from build123d import *

# Parameters (mm, degrees)
SKETCH_R        = 11.3
SKETCH_R_2      = 1.6
SKETCH_R_3      = 3.2
PAD_DEPTH       = 15
SKETCH001_R     = 3.2
POCKET_DEPTH    = 3.4
SKETCH002_R     = 6.1
POCKET001_DEPTH = 4
FILLET_R        = 4
FILLET001_R     = 4
CHAMFER_SIZE    = 0.6
CHAMFER001_SIZE = 0.6
CHAMFER002_SIZE = 0.6


with BuildPart() as part:
    # Sketch → Pad (new body)
    with BuildSketch(Plane.XY):
        Polygon((20, 30), (20, 58), (62.3, 58), (62.3, 30), (82.3, 30), (82.3, 0), (0, 0), (0, 30), align=None)
        with Locations((41.15, 36.85)):
            Circle(SKETCH_R, mode=Mode.SUBTRACT)
        with Locations((25.65, 52.35)):
            Circle(SKETCH_R_2, mode=Mode.SUBTRACT)
        with Locations((25.65, 21.35)):
            Circle(SKETCH_R_2, mode=Mode.SUBTRACT)
        with Locations((56.65, 52.35)):
            Circle(SKETCH_R_2, mode=Mode.SUBTRACT)
        with Locations((56.65, 21.35)):
            Circle(SKETCH_R_2, mode=Mode.SUBTRACT)
        with Locations((11.15, 10)):
            Circle(SKETCH_R_3, mode=Mode.SUBTRACT)
        with Locations((31.15, 10)):
            Circle(SKETCH_R_3, mode=Mode.SUBTRACT)
        with Locations((51.15, 10)):
            Circle(SKETCH_R_3, mode=Mode.SUBTRACT)
        with Locations((71.15, 10)):
            Circle(SKETCH_R_3, mode=Mode.SUBTRACT)
    extrude(amount=PAD_DEPTH)

    # Sketch001 (on Face19 of Pad) → Pocket (cut)
    with BuildSketch(Plane.XY.offset(15)):
        with Locations((25.65, 52.35)):
            Circle(SKETCH001_R)
        with Locations((56.65, 52.35)):
            Circle(SKETCH001_R)
        with Locations((56.65, 21.35)):
            Circle(SKETCH001_R)
        with Locations((25.65, 21.35)):
            Circle(SKETCH001_R)
    extrude(amount=-POCKET_DEPTH, mode=Mode.SUBTRACT)

    # Sketch002 (on Face4 of Pocket) → Pocket001 (cut)
    with BuildSketch(Plane(origin=(0, 0, 0), x_dir=(1, 0, 0), z_dir=(0, 0, -1))):
        with Locations((11.15, -10)):
            Circle(SKETCH002_R)
        with Locations((31.15, -10)):
            Circle(SKETCH002_R)
        with Locations((51.15, -10)):
            Circle(SKETCH002_R)
        with Locations((71.15, -10)):
            Circle(SKETCH002_R)
    extrude(amount=-POCKET001_DEPTH, mode=Mode.SUBTRACT)

    # Fillet
    fillet_edges = [part.edges().sort_by_distance(p)[0] for p in [
        (0, 30, 7.5),
        (20, 58, 7.5),
        (62.3, 58, 7.5),
        (82.3, 30, 7.5),
        (0, 0, 7.5),
        (82.3, 0, 7.5),
    ]]
    fillet(fillet_edges, radius=FILLET_R)

    # Fillet001
    fillet001_edges = [part.edges().sort_by_distance(p)[0] for p in [
        (20, 30, 7.5),
        (62.3, 30, 7.5),
    ]]
    fillet(fillet001_edges, radius=FILLET001_R)

    # Chamfer
    chamfer_edges = [part.edges().sort_by_distance(p)[0] for p in [
        (20, 44, 0),
        (18.828427, 31.171573, 0),
        (21.171573, 56.828427, 0),
        (10, 30, 0),
        (41.15, 58, 0),
        (1.171573, 28.828427, 0),
        (61.128427, 56.828427, 0),
        (0, 15, 0),
        (62.3, 44, 0),
        (1.171573, 1.171573, 0),
        (63.471573, 31.171573, 0),
        (41.15, 0, 0),
        (72.3, 30, 0),
        (81.128427, 1.171573, 0),
        (81.128427, 28.828427, 0),
        (82.3, 15, 0),
        (29.85, 36.85, 0),
        (55.05, 52.35, 0),
        (24.05, 52.35, 0),
        (25.05, 10, 0),
        (24.05, 21.35, 0),
        (55.05, 21.35, 0),
        (45.05, 10, 0),
        (65.05, 10, 0),
        (5.05, 10, 0),
    ]]
    chamfer(chamfer_edges, length=CHAMFER_SIZE)

    # Chamfer001
    chamfer001_edges = [part.edges().sort_by_distance(p)[0] for p in [
        (20, 44, 15),
        (18.828427, 31.171573, 15),
        (21.171573, 56.828427, 15),
        (10, 30, 15),
        (41.15, 58, 15),
        (1.171573, 28.828427, 15),
        (61.128427, 56.828427, 15),
        (0, 15, 15),
        (62.3, 44, 15),
        (1.171573, 1.171573, 15),
        (63.471573, 31.171573, 15),
        (41.15, 0, 15),
        (72.3, 30, 15),
        (81.128427, 1.171573, 15),
        (81.128427, 28.828427, 15),
        (82.3, 15, 15),
        (29.85, 36.85, 15),
        (53.45, 52.35, 15),
        (53.45, 21.35, 15),
        (67.95, 10, 15),
        (47.95, 10, 15),
        (27.95, 10, 15),
        (22.45, 21.35, 15),
        (22.45, 52.35, 15),
        (7.95, 10, 15),
    ]]
    chamfer(chamfer001_edges, length=CHAMFER001_SIZE)

    # Chamfer002
    chamfer002_edges = [part.edges().sort_by_distance(p)[0] for p in [
        (67.95, 10, 4),
        (47.95, 10, 4),
        (27.95, 10, 4),
        (7.95, 10, 4),
    ]]
    chamfer(chamfer002_edges, length=CHAMFER002_SIZE)


solid = part.part
Design review of the part built by this model. Coordinates are the model's own, in mm. A direction names the side the tool comes from. Round coordinates to 2 decimals unless told otherwise and drop trailing zeros. Order: outer loops, then holes, each group sorted by start corner. A loop starts at its lowest first (then second) coordinate and runs counter-clockwise, first axis right, second up. Notation, with made-up numbers: M -31.5,-35.75 L -11.5,-35.75 A18 cw -11.5,-9.75 Z; hole C 33.5,-13.5 d3. An arc over 180 degrees is marked long. Answer as CSV lines item,"result". Start each with the question number.
1) Tool access review of faces 4 (the face through (58.176, 21.831, 6.023)), 5 (the face through (28.702, 22.311, 13.02)), 6 (the face through (56.8, 12.3, 2.3)): name each direction out of +Z, -Z, +X, -X, +Y, -Y from which nothing blocks a thin tool from reaching the whole face with its end or side.
2) The part is to be moulded in two halves that separate along X. For faces 1 (the face through (1.141, 1.203, 7.597)), 2 (the face through (9.828, 15.955, 2.276)), 3 (the face through (80.791, 28.547, 0.162)), say which applies: +X half, -X half, draft (parallel to the pull), parting line (faces both ways), or undercut.
3) For pin 1 Ø6 at (x, y) = (49, 12.5) entering from -Z; pin 2 Ø14 at (x, y) = (51.15, 10) entering from -Z; pin 3 Ø4 at (y, z) = (46.5, 4) entering from +X; pin 4 Ø7.5 at (x, y) = (71.15, 10) entering from -Z, all flat-tipped, find the tip position at first contact; note any pin that passes through.
4) Add section A-A (y = 52.35). Give the number of separate pieces and of enclosed holes in the cut face, then the cut area to 3 significant figures.
5) Wall thickness on line 1 along X through (y, z) = (10, 2.75); line 2 along X through (y, z) = (10, 10.5); line 3 along Y through (x, z) = (25.65, 7.25): over which ranges is each line inside the solid? List them lowest first. Write a range as [from, to].
6) Add section C-C (x = 71.15). Give the boundary of the cut face in (y, z).
Resolved:
1,face 4,"+Z, -Z"
1,face 5,"+Z"
1,face 6,"-Z"
2,face 1,"-X half"
2,face 2,"undercut"
2,face 3,"+X half"
3,pin 1,"z = 0.4"
3,pin 2,"z = 0"
3,pin 3,"x = 62.3"
3,pin 4,"z = 4.05"
4,separate pieces,"3"
4,enclosed holes,"0"
4,area,"515 mm^2"
5,line 1,"[0, 5.05], [17.25, 25.05], [37.25, 45.05], [57.25, 65.05], [77.25, 82.3]"
5,line 2,"[0, 7.95], [14.35, 27.95], [34.35, 47.95], [54.35, 67.95], [74.35, 82.3]"
5,line 3,"[0, 19.75], [22.95, 50.75], [53.95, 58]"
6,outline,"M 0,0.6 L 0.6,0 L 3.3,0 L 3.9,0.6 L 3.9,4 L 6.2,4 L 6.8,4.6 L 6.8,14.4 L 6.2,15 L 0.6,15 L 0,14.4 Z; M 13.2,4.6 L 13.8,4 L 16.1,4 L 16.1,0.6 L 16.7,0 L 29.4,0 L 30,0.6 L 30,14.4 L 29.4,15 L 13.8,15 L 13.2,14.4 Z"
